The drawing under review shows one solid part. Ordinate dimensions are in mm from its lowest x, y, z. A direction names the side the tool comes from. Coordinates: 2 decimals unless noted, no trailing zeros. Write each loop counter-clockwise with the first axis right and the second up, starting at its lowest first coordinate (ties: lowest second). Pieces come first, ordered by that corner, then holes. Notation, with made-up numbers: M 16,69.5 L 37,69.5 A12 ccw 37,80.5 Z; hole C 5.5,-31 d3. An arc over 180 degrees is marked long. Write item = value, one per line.
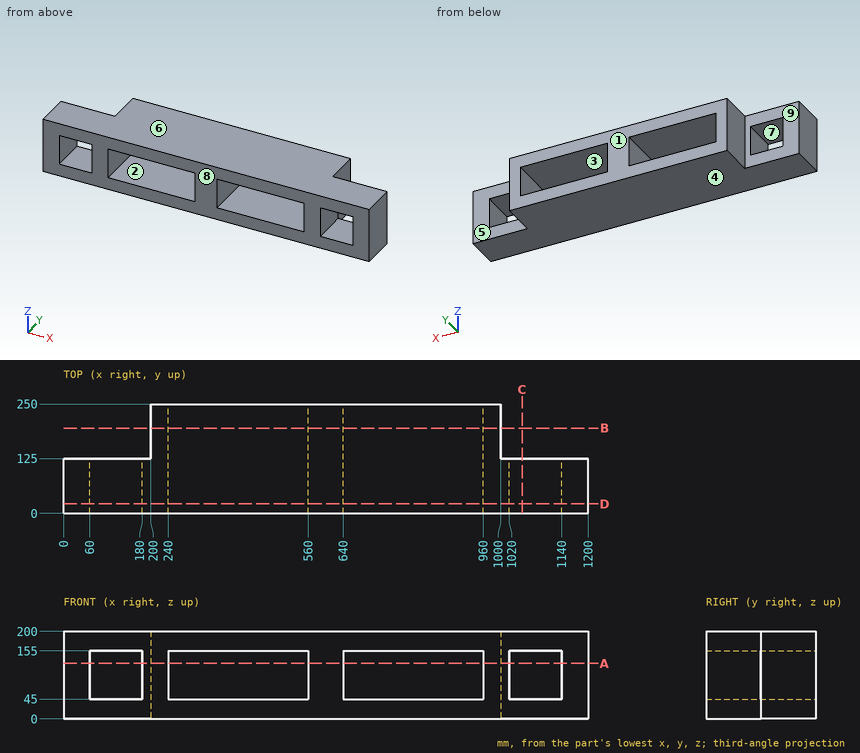
Q1. For P1, Ø5, axis at y = 221.5, z = 158, coming from the +X side, flat-tipped, find the tip position at first contact; note if it passes through.
Check result:
P1 = 1000
Q2. Consider section A-A, the plane z = 126.5. State the section outline as (x, y) points.
Check result:
outline = M 0,0 L 60,0 L 60,125 L 0,125 Z; M 180,0 L 240,0 L 240,250 L 200,250 L 200,125 L 180,125 Z; M 560,0 L 640,0 L 640,250 L 560,250 Z; M 960,0 L 1020,0 L 1020,125 L 1000,125 L 1000,250 L 960,250 Z; M 1140,0 L 1200,0 L 1200,125 L 1140,125 Z
Q3. Machinability: for the marked faces 5, 6, 7, 8 and 9, which of the approach directions +Z, -Z, +X, -X, +Y, -Y give a long, thin tool a straight path to every point of the face, cutting with its end or side? Answer none if there is none.
Check result:
face_5 = +Z, -Z, +X, +Y
face_6 = +Z, +X, -X, +Y, -Y
face_7 = +Y, -Y
face_8 = +Z, -Z, +X, -X, -Y
face_9 = +Z, -Z, -X, +Y
Q4. Consider section C-C, the plane x = 1049. State the section outline as (y, z) points.
Check result:
outline = M 0,0 L 125,0 L 125,45 L 0,45 Z; M 0,155 L 125,155 L 125,200 L 0,200 Z
Q5. The part is to be moulded in two halves that separate along Z. For the marked faces 1, 2, 3 and 4, say which applies: +Z half, -Z half, draft (parallel to the pull), parting line (faces both ways), or undercut.
Check result:
face_1 = draft
face_2 = undercut
face_3 = undercut
face_4 = -Z half
Q6. Consider section B-B, the plane y = 195. State the section outline as (x, z) points, and give its area (3 significant figures).
Check result:
outline = M 200,0 L 1000,0 L 1000,200 L 200,200 Z; hole M 240,45 L 560,45 L 560,155 L 240,155 Z; hole M 640,45 L 960,45 L 960,155 L 640,155 Z
area = 89,600 mm²
Q7. Wall thickness on line 1 (X direction, y = 119, z = 79); line 2 (Z direction, x = 254, y = 51.5); line 3 (X direction, y = 153, z = 69.5): over which ranges is each line inside the solid? List them lowest first.
Check result:
line_1 = 0 to 60, 180 to 240, 560 to 640, 960 to 1020, 1140 to 1200
line_2 = 0 to 45, 155 to 200
line_3 = 200 to 240, 560 to 640, 960 to 1000
Q8. Consider section D-D, the plane y = 21.5. State the section outline as (x, z) points, and give its area (3 significant figures).
Check result:
outline = M 0,0 L 1200,0 L 1200,200 L 0,200 Z; hole M 60,45 L 180,45 L 180,155 L 60,155 Z; hole M 240,45 L 560,45 L 560,155 L 240,155 Z; hole M 640,45 L 960,45 L 960,155 L 640,155 Z; hole M 1020,45 L 1140,45 L 1140,155 L 1020,155 Z
area = 143,000 mm²
